The listing builds one solid part. Answer for the finished solid, in the listing's coordinates (mm). A direction names the side the tool comes from. Give positions to 0.01 mm unless a question says otherwise; leave off trailing zeros. Order: outer loops, then holes, each group sorted by start corner. A loop starts at its lowest first (then second) coordinate and runs counter-clockwise, first axis right, second up. Notation, with made-up numbers: (86, -29.5) - (139, -29.5) arc R26 cw to (139, -6.5) - close; hole circle Ø7 at (43, -36). An arc over 180 degrees is marked (long way). Use a Markdown table: item, result. Add a question column.
1) Find section A-A, the plane x = 15. Determine the outline of the cut face in (y, z), plus the area to 3 significant figures.
2) Find section B-B, the plane y = 2.9. Determine the outline of the cut face in (x, z).
3) Straight lines are drawn through the part: line 1 (X direction, y = 4.95, z = 14); line 2 (X direction, y = 1.4, z = 0); line 3 (X direction, y = 4.5, z = 0). For each, find the intervals that lie inside material, in ascending order.
4) The mould has two halves that part along X. Classify faces 4 (the face through (30, 1, -36)), 5 (the face through (38, 3, 39)), 6 (the face through (-16.1, 4, 0)), 7 (the face through (-39, 3, -38)): released by +X, released by -X, zero draft, split by the parting line, or undercut.
5) A flat-ended cylindrical pin translates along its axis: pin 1 (4 mm diameter, centred on x = 0, z = 0, fed in from +Y). Find the tip coordinate at first contact, or state that the pin passes through.
6) Find section D-D, the plane x = 0. Determine the outline of the cut face in (y, z), plus the area to 3 significant figures.
7) For faces 1 (the face through (-39, 3, 38)), 2 (the face through (-13.6, 1.8, -0.5)), 3 (the face through (-28.9, 4, 0)), determine the directions among +Z, -Z, +X, -X, +Y, -Y from which every point of the face is accessible in a straight line to the end or side of a thin tool.
8) Find section C-C, the plane z = 0. State how many separate pieces and enclosed holes the cut face has, plus the area to 3 significant figures.
from build123d import *

# Parameters (mm, degrees)
SKETCH1_W            = 80
SKETCH1_H            = 80
BOSS_EXTRUDE1_DEPTH  = 6
CUT_EXTRUDE1_DEPTH   = 57.885850613
CUT_EXTRUDE2_DEPTH   = 1.8
LPATTERN1_COUNT      = 2
LPATTERN1_PITCH      = 15
MIRROR1_COPY_1_DEPTH = 57.885850613
MIRROR1_COPY_2_DEPTH = 1.8
SKETCH5_R            = 3.5
CUT_EXTRUDE3_DEPTH   = 4
SKETCH6_R            = 2.1
CUT_EXTRUDE4_DEPTH   = 57.709787515
FILLET3_R            = 5


with BuildPart() as part:
    # Sketch1 → Boss-Extrude1 (new body)
    with BuildSketch(Plane(origin=(0, 0, 0), x_dir=(1, 0, 0), z_dir=(0, 1, 0))):
        Rectangle(SKETCH1_W, SKETCH1_H)
    extrude(amount=BOSS_EXTRUDE1_DEPTH)

    # Sketch2 → Cut-Extrude1 (cut, through all)
    with BuildSketch(Plane(origin=(0, 6, 0), x_dir=(1, 0, 0), z_dir=(0, 1, 0))):
        with BuildLine():
            Line((16.1, 34), (16.1, -34))
            ThreePointArc((16.1, -34), (15, -35.1), (13.9, -34))
            Line((13.9, -34), (13.9, 34))
            ThreePointArc((13.9, 34), (15, 35.1), (16.1, 34))
        make_face()
    cut_extrude1 = extrude(amount=-CUT_EXTRUDE1_DEPTH, mode=Mode.SUBTRACT)

    # Sketch4 → Cut-Extrude2 (cut)
    with BuildSketch(Plane(origin=(0, 0, 0), x_dir=(1, 0, 0), z_dir=(0, 1, 0))):
        with BuildLine():
            Line((13, 34), (13, -34))
            ThreePointArc((13, -34), (15, -36), (17, -34))
            Line((17, -34), (17, 34))
            ThreePointArc((17, 34), (15, 36), (13, 34))
        make_face()
    cut_extrude2 = extrude(amount=CUT_EXTRUDE2_DEPTH, mode=Mode.SUBTRACT)

    # LPattern1: Cut-Extrude1, Cut-Extrude2 ×2
    with Locations(*[(i * LPATTERN1_PITCH, 0, 0) for i in range(1, LPATTERN1_COUNT)]):
        add(cut_extrude1, mode=Mode.SUBTRACT)
        add(cut_extrude2, mode=Mode.SUBTRACT)

    # Mirror1: Cut-Extrude1, Cut-Extrude2 across plane
    add(cut_extrude1.mirror(Plane(origin=(0, 0, 0), x_dir=(0, 0, 1), z_dir=(1, 0, 0))), mode=Mode.SUBTRACT)
    add(cut_extrude2.mirror(Plane(origin=(0, 0, 0), x_dir=(0, 0, 1), z_dir=(1, 0, 0))), mode=Mode.SUBTRACT)

    # Mirror1 copy 1 sketch → Mirror1 copy 1 (cut, through all)
    with BuildSketch(Plane(origin=(-15, 6, 0), x_dir=(-1, 0, 0), z_dir=(0, 1, 0))):
        with BuildLine():
            Line((16.1, -34), (16.1, 34))
            ThreePointArc((16.1, 34), (15, 35.1), (13.9, 34))
            Line((13.9, 34), (13.9, -34))
            ThreePointArc((13.9, -34), (15, -35.1), (16.1, -34))
        make_face()
    extrude(amount=-MIRROR1_COPY_1_DEPTH, mode=Mode.SUBTRACT)

    # Mirror1 copy 2 sketch → Mirror1 copy 2 (cut)
    with BuildSketch(Plane(origin=(-15, 0, 0), x_dir=(-1, 0, 0), z_dir=(0, 1, 0))):
        with BuildLine():
            Line((13, -34), (13, 34))
            ThreePointArc((13, 34), (15, 36), (17, 34))
            Line((17, 34), (17, -34))
            ThreePointArc((17, -34), (15, -36), (13, -34))
        make_face()
    extrude(amount=MIRROR1_COPY_2_DEPTH, mode=Mode.SUBTRACT)

    # Sketch5 → Cut-Extrude3 (cut)
    with BuildSketch(Plane.XZ.offset(-6)):
        with Locations(Location((0, 0, 0), (0, 0, 270))):
            Circle(SKETCH5_R)
    extrude(amount=CUT_EXTRUDE3_DEPTH, mode=Mode.SUBTRACT)

    # Sketch6 → Cut-Extrude4 (cut, through all)
    with BuildSketch(Plane(origin=(0, 2, 0), x_dir=(1, 0, 0), z_dir=(0, 1, 0))):
        with Locations(Location((0, 0, 0), (0, 0, 270))):
            Circle(SKETCH6_R)
    extrude(amount=-CUT_EXTRUDE4_DEPTH, mode=Mode.SUBTRACT)

    # Fillet3
    fillet3_edges = [part.edges().sort_by_distance(p)[0] for p in [
        (40, 3, 40),
        (-40, 3, 40),
        (-40, 3, -40),
        (40, 3, -40),
    ]]
    fillet(fillet3_edges, radius=FILLET3_R)


solid = part.part
The answers:
| question | item | result |
|---|---|---|
| 1 | outline | (0, -40) - (6, -40) - (6, -35.1) - (1.8, -35.1) - (1.8, -36) - (0, -36) - close; (0, 36) - (1.8, 36) - (1.8, 35.1) - (6, 35.1) - (6, 40) - (0, 40) - close |
| 1 | area | 55.6 mm2 |
| 2 | outline | (-40, -35) arc R5 ccw to (-35, -40) - (35, -40) arc R5 ccw to (40, -35) - (40, 35) arc R5 ccw to (35, 40) - (-35, 40) arc R5 ccw to (-40, 35) - close; hole (-31.1, -34) arc R1.1 ccw to (-28.9, -34) - (-28.9, 34) arc R1.1 ccw to (-31.1, 34) - close; hole (-16.1, -34) arc R1.1 ccw to (-13.9, -34) - (-13.9, 34) arc R1.1 ccw to (-16.1, 34) - close; hole circle Ø7 at (0, 0); hole (13.9, -34) arc R1.1 ccw to (16.1, -34) - (16.1, 34) arc R1.1 ccw to (13.9, 34) - close; hole (28.9, -34) arc R1.1 ccw to (31.1, -34) - (31.1, 34) arc R1.1 ccw to (28.9, 34) - close |
| 3 | line 1 | -40 to -31.1, -28.9 to -16.1, -13.9 to 13.9, 16.1 to 28.9, 31.1 to 40 |
| 3 | line 2 | -40 to -32, -28 to -17, -13 to -2.1, 2.1 to 13, 17 to 28, 32 to 40 |
| 3 | line 3 | -40 to -31.1, -28.9 to -16.1, -13.9 to -3.5, 3.5 to 13.9, 16.1 to 28.9, 31.1 to 40 |
| 4 | face 4 | undercut |
| 4 | face 5 | released by +X |
| 4 | face 6 | undercut |
| 4 | face 7 | released by -X |
| 5 | pin 1 | through |
| 6 | outline | (0, -40) - (6, -40) - (6, -3.5) - (2, -3.5) - (2, -2.1) - (0, -2.1) - close; (0, 2.1) - (2, 2.1) - (2, 3.5) - (6, 3.5) - (6, 40) - (0, 40) - close |
| 6 | area | 444 mm2 |
| 7 | face 1 | +Z, -X, +Y, -Y |
| 7 | face 2 | -Y |
| 7 | face 3 | +Y, -Y |
| 8 | separate pieces | 6 |
| 8 | enclosed holes | 0 |
| 8 | area | 378 mm2 |
